```python
from build123d import *

# Parameters (mm, degrees)
SKETCH1_R           = 4
SKETCH1_R_2         = 3.45
BOSS_EXTRUDE1_DEPTH = 3
FILLET1_R           = 5
FILLET2_R           = 10


with BuildPart() as part:
    # Sketch1 → Boss-Extrude1 (new body)
    with BuildSketch(Plane(origin=(0, 0, 0), x_dir=(1, 0, 0), z_dir=(0, 1, 0))):
        with BuildLine():
            Line((-15, -325), (-15, -345))
            Line((-15, -345), (45, -345))
            Line((45, -345), (45, -325))
            add(Edge.make_bspline(
                [(83.906024568, -72.334193472), (100.067703513, -103.783632704), (75.99628029, -191.959172621), (49.567481947, -271.364145728), (45, -325)],
                knots=[0, 0, 0, 0, 0.388668159, 1, 1, 1, 1], degree=3))
            add(Edge.make_bspline(
                [(0, 15), (11.859468256, 15), (19.027998929, 4.991144095), (28.068840843, -60.357487218), (48.218476882, -67.479548025), (83.906024568, -72.334193472)],
                knots=[0, 0, 0, 0, 0.292385063, 0.473698528, 1, 1, 1, 1], degree=3))
            Line((0, 15), (-30, 15))
            add(Edge.make_bspline(
                [(-30, 15), (-42.027894854, -69.718453242), (-28.647636574, -182.406317953), (-15, -295.84878712), (-15, -325)],
                knots=[0, 0, 0, 0, 0.742442908, 1, 1, 1, 1], degree=3))
        make_face()
        Circle(SKETCH1_R, mode=Mode.SUBTRACT)
        with Locations((47.5, -226.5)):
            Circle(SKETCH1_R_2, mode=Mode.SUBTRACT)
        with BuildLine():
            Line((-13.48245603, -250.35), (-23.48245603, -150.851256289))
            ThreePointArc((-23.48245603, -150.851256289), (-20.35, -147.018800259), (-16.51754397, -150.151256289))
            Line((-16.51754397, -150.151256289), (-6.51754397, -249.65))
            ThreePointArc((-6.51754397, -249.65), (-9.65, -253.48245603), (-13.48245603, -250.35))
        make_face(mode=Mode.SUBTRACT)
    extrude(amount=BOSS_EXTRUDE1_DEPTH)

    # Fillet1
    fillet1_edges = [part.edges().sort_by_distance(p)[0] for p in [
        (83.906024568, 1.5, 72.334193472),
        (45, 1.5, 345),
        (-15, 1.5, 345),
    ]]
    fillet(fillet1_edges, radius=FILLET1_R)

    # Fillet2
    fillet2_edges = [part.edges().sort_by_distance(p)[0] for p in [
        (-30, 1.5, -15),
    ]]
    fillet(fillet2_edges, radius=FILLET2_R)


solid = part.part
```
Geometry: final body of the model. Coordinates: model frame, mm. A direction names the side the tool comes from. Coordinates: 2 decimals unless noted, no trailing zeros. Answer in a Markdown table with one row per item. Add a question column.
Q1. Section query A-A on y = 1.6. Count the separate pieces of the cut face and the enclosed holes in it, and give its area (3 significant figures).
Q2. Contact query for flat-ended pins moving along their axis: P1, Ø3, axis at x = 57, z = 264, coming from the +Y side; P2, Ø0.9, axis at y = 1, z = 334, coming from the -X side; P3, Ø0.9, axis at y = 1, z = 331.5, coming from the +X side. Output: stop coordinate, or through.
Q3. Line query: L1, parallel to Z at x = 0, y = 1.25; L2, parallel to X at y = 1.5, z = 226.5; L3, parallel to X at y = 0.4, z = 326. Output: solid intervals per line, ascending.
Q4. Reachability of faces 3 (the flat face through (-18.412, 1.479, 201.297)), 4 (the flat face through (28, 0, 162)) from +Z, -Z, +X, -X, +Y, -Y: full face, straight path, thin tool, end or side. Return the list, or none.
Q5. Mould query, pull axis X, two halves, no side actions, for faces 1 (the flat face through (-11.588, 1.479, 199.204)), 2 (the flat face through (28, 3, 162)). Classes: released by +X, released by -X, zero draft, split by the parting line, or undercut.
Completed:
| question | item | result |
|---|---|---|
| 1 | separate pieces | 1 |
| 1 | enclosed holes | 3 |
| 1 | area | 30,400 mm2 |
| 2 | P1 | passes through |
| 2 | P2 | stops at x = -15 |
| 2 | P3 | stops at x = 45 |
| 3 | L1 | z = -15 to -4, 4 to 345 |
| 3 | L2 | x = -23.32 to -15.88, -8.84 to 44.05, 50.95 to 64.62 |
| 3 | L3 | x = -15 to 45 |
| 4 | face 3 | +Y, -Y |
| 4 | face 4 | +Z, -Z, +X, -X, -Y |
| 5 | face 1 | undercut |
| 5 | face 2 | zero draft |
